Input: part model. Units: mm. Frame: model coordinates. Face numbers are marked on the shaded views. A direction names the side the tool comes from. Give positions to 0.01 mm unless a question says otherwise; leave off trailing zeros. Loops run counter-clockwise (first coordinate to the right, second up) from the corner with the lowest first, then second, coordinate; pieces in that order, holes last. Notation, with made-up numbers: M 33.25,27 L 83.25,27 A23 ccw 83.25,66 Z; hole C -22,65 d2. An arc over 180 degrees is marked long. Answer as a JSON object with one key per item and string values. Group by question number.
```python
from build123d import *

# Parameters (mm, degrees)
SKETCH2_R           = 1.9
SKETCH2_R_2         = 3.4
BOSS_EXTRUDE1_DEPTH = 4
SKETCH3_R           = 0.6
CUT_EXTRUDE1_DEPTH  = 6
FILLET1_R           = 3


with BuildPart() as part:
    # Sketch2 → Boss-Extrude1 (new body)
    with BuildSketch(Plane(origin=(0, 0, 0), x_dir=(1, 0, 0), z_dir=(0, 1, 0))):
        with BuildLine():
            ThreePointArc((49.0624911, 100.728722197), (55.253975507, 111.876765002), (45.278809785, 103.932622106))
            Line((45.278809785, 103.932622106), (41.677103445, 98.359455452))
            Line((41.677103445, 98.359455452), (40.917682236, 97.184351056))
            ThreePointArc((40.917682236, 97.184351056), (40.000914232, 93.684113367), (40.729811239, 90.139986308))
            Line((40.729811239, 90.139986308), (51.995593872, 69.121735128))
            Line((51.995593872, 69.121735128), (52.448751423, 68.276291936))
            ThreePointArc((52.448751423, 68.276291936), (53.733769558, 66.46917356), (55.737555004, 65.519546097))
            Line((55.737555004, 65.519546097), (56.575581952, 65.474059755))
            Line((56.575581952, 65.474059755), (56.904280571, 65.456218685))
            Line((56.904280571, 65.456218685), (64.043852088, 65.068697747))
            Line((64.043852088, 65.068697747), (67.659658755, 64.927019071))
            ThreePointArc((67.659658755, 64.927019071), (68.973857559, 62.514332624), (71.364365032, 61.16020988))
            Line((71.364365032, 61.16020988), (77.3922419, 49.235496946))
            ThreePointArc((77.3922419, 49.235496946), (85.295038859, 43.696471142), (81.278467798, 52.471558808))
            Line((81.278467798, 52.471558808), (75.926202221, 62.342787356))
            ThreePointArc((75.926202221, 62.342787356), (77.117833046, 64.012589982), (77.538655529, 66.020358214))
            Line((77.538655529, 66.020358214), (73.882441794, 69.676571949))
            Line((73.882441794, 69.676571949), (69.341583584, 69.864669723))
            Line((69.341583584, 69.864669723), (65.404712603, 69.864669723))
            Line((65.404712603, 69.864669723), (58.04793187, 69.864669723))
            ThreePointArc((58.04793187, 69.864669723), (56.992330015, 70.157110244), (56.212176606, 70.925990854))
            ThreePointArc((56.212176606, 70.925990854), (56.161986001, 71.014595828), (56.115987655, 71.105447853))
            Line((56.115987655, 71.105447853), (45.913475043, 90.139986308))
            ThreePointArc((45.913475043, 90.139986308), (45.708651409, 90.489699119), (45.530826332, 90.853883157))
            ThreePointArc((45.530826332, 90.853883157), (45.074746145, 93.175228741), (45.661998303, 95.466907026))
            Line((45.661998303, 95.466907026), (49.0624911, 100.728722197))
        make_face()
        with Locations(Location((82.095552315, 47.538773298, 0), (0, 0, 270))):
            Circle(SKETCH2_R, mode=Mode.SUBTRACT)
        with Locations(Location((72.538655529, 66.020358214, 0), (0, 0, 270))):
            Circle(SKETCH2_R, mode=Mode.SUBTRACT)
        with Locations(Location((51.053576092, 106.916256485, 0), (0, 0, 270))):
            Circle(SKETCH2_R_2, mode=Mode.SUBTRACT)
    extrude(amount=BOSS_EXTRUDE1_DEPTH)

    # Sketch3 → Cut-Extrude1 (cut)
    with BuildSketch(Plane(origin=(0, 4, 0), x_dir=(1, 0, 0), z_dir=(0, 1, 0))):
        with Locations(Location((42.353398584, 95.378951282, 0), (0, 0, 270))):
            Circle(SKETCH3_R)
        with Locations(Location((43.557575402, 96.975810134, 0), (0, 0, 270))):
            Circle(SKETCH3_R)
        with Locations(Location((44.761752219, 98.572668985, 0), (0, 0, 270))):
            Circle(SKETCH3_R)
        with Locations(Location((45.965929037, 100.169527837, 0), (0, 0, 270))):
            Circle(SKETCH3_R)
    extrude(amount=-CUT_EXTRUDE1_DEPTH, mode=Mode.SUBTRACT)

    # Fillet1
    fillet1_edges = [part.edges().sort_by_distance(p)[0] for p in [
        (71.364365032, 2, -61.16020988),
        (67.659658755, 2, -64.927019071),
        (45.278809785, 2, -103.932622106),
        (49.0624911, 2, -100.728722197),
        (73.882441794, 2, -69.676571949),
        (77.538655529, 2, -66.020358214),
        (75.926202221, 2, -62.342787356),
        (81.278467798, 2, -52.471558808),
        (77.3922419, 2, -49.235496946),
    ]]
    fillet(fillet1_edges, radius=FILLET1_R)


solid = part.part
```
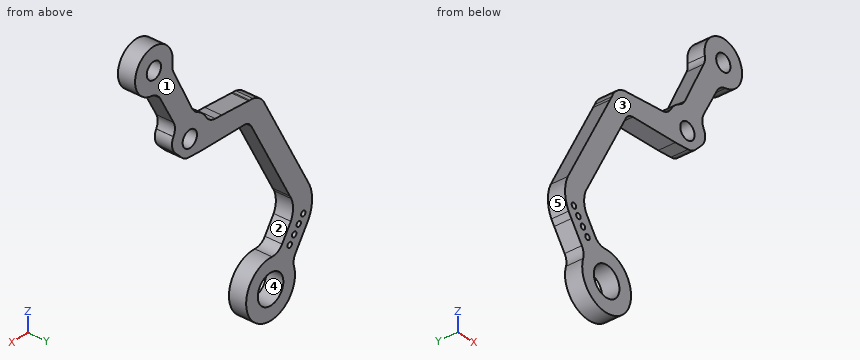
1. Material intervals for L1, parallel to Z at x = 48, y = 2.8; L2, parallel to Z at x = 49.5, y = 3.25; L3, parallel to X at y = 0.55, z = -93, sorted ascending.
2. Section D-D (x = 62). Output: boundary loops of the cut face in (y, z), then the cut area to 3 significant figures.
3. Section A-A (z = -107.5). Output: boundary loops of the cut face in (x, y), then the cut area to 3 significant figures.
4. Reachability of the marked faces 1 and 2 from +Z, -Z, +X, -X, +Y, -Y: full face, straight path, thin tool, end or side. Return the list, or none.
5. Section B-B (z = -84.5). Output: boundary loops of the cut face in (x, y), then the cut area to 3 significant figures.
6. Mould query, pull axis Z, two halves, no side actions, for the marked faces 3, 4 and 5. Classes: pulls with the +Z half, pulls with the -Z half, needs draft (parallel to the pull), parting line crosses it, or undercut.
7. First-contact query: P1, Ø1.2, axis at x = 66, y = 1.5, coming from the -Z side; P2, Ø1.5, axis at y = 1, z = -64.5, coming from the +X side. Flat tips, straight axial feed; report the tip coordinate or a pass-through.
8. Section C-C (y = 0.65). Count the separate pieces of the cut face and the enclosed holes in it, then the cut area to 3 significant figures.
Geometry results:
{
 "1": {"L1": "-112.65 to -108.41, -105.42 to -99.08, -86.25 to -76.58", "L2": "-113.23 to -109.94, -103.89 to -100.26, -83.45 to -73.78", "L3": "40.01 to 45.07"},
 "2": {"outline": "M 0,-69.86 L 4,-69.86 L 4,-65.18 L 0,-65.18 Z", "area": "18.7 mm2"},
 "3": {"outline": "M 44.58,0 L 47.7,0 L 47.7,4 L 44.58,4 Z; M 54.4,0 L 57.53,0 L 57.53,4 L 54.4,4 Z", "area": "25.0 mm2"},
 "4": {"face 1": "+Z, -Z, +X, -X, +Y", "face 2": "+X, +Y, -Y"},
 "5": {"outline": "M 43.75,0 L 48.94,0 L 48.94,4 L 43.75,4 Z", "area": "20.7 mm2"},
 "6": {"face 3": "needs draft", "face 4": "undercut", "face 5": "parting line crosses it"},
 "7": {"P1": "z = -69.86", "P2": "x = 77.28"},
 "8": {"separate pieces": "1", "enclosed holes": "7", "area": "512 mm2"}
}
